Geometry: final body of the model. Coordinates: model frame, mm. A direction names the side the tool comes from. Give positions to 0.01 mm unless a question says otherwise; leave off trailing zeros. Write each loop counter-clockwise with the first axis right and the second up, starting at its lowest first coordinate (ties: lowest second). Pieces come first, ordered by that corner, then holes.
```python
from build123d import *

# Parameters (mm, degrees)
FILLET2_R      = 6
CHAMFER1_SIZE  = 1
CHAMFER1_SIZE2 = 2
CHAMFER2_SIZE  = 0.5


with BuildPart() as part:
    # Sketch1 → Revolve1 (revolve)
    with BuildSketch(Plane(origin=(0, 0, 0), x_dir=(0, 0, -1), z_dir=(1, 0, 0))):
        Polygon((0, 0), (0, -80), (11, -80), (11, -77), (2.5, -77), (2.5, -8), (1.5, -8), (1.5, -3), (2.5, -3), (2.5, 0), align=None)
    revolve(axis=Axis((0, 0, 0), (0, -1, 0)))

    # Fillet2
    fillet2_edges = [part.edges().sort_by_distance(p)[0] for p in [
        (0, -77, 2.5),
    ]]
    fillet(fillet2_edges, radius=FILLET2_R)

    # Chamfer1
    chamfer1_edges = [part.edges().sort_by_distance(p)[0] for p in [
        (0, -77, 11),
    ]]
    chamfer1_side = [part.faces().sort_by_distance(p)[0] for p in [
        (0, -78.5, 11),
    ]]
    chamfer(chamfer1_edges, length=CHAMFER1_SIZE, length2=CHAMFER1_SIZE2, reference=chamfer1_side[0])

    # Chamfer2
    chamfer2_edges = [part.edges().sort_by_distance(p)[0] for p in [
        (0, 0, 2.5),
    ]]
    chamfer(chamfer2_edges, length=CHAMFER2_SIZE)


solid = part.part
```
Item 1: Pull-direction query (Y, two-part tool) for faces 4 (the face through (0, -3, 2)), 5 (the face through (-2.44, -1.73, 0.54)), 6 (the face through (0, 0, 0)); classes: +Y half, -Y half, draft (parallel to the pull), parting line (faces both ways), or undercut.
Found:
face 4: undercut
face 5: draft
face 6: +Y half
Item 2: Section A-A, the plane x = 0. Return the cut outline in (y, z).
Found:
outline: (-80, -11) - (-78, -11) - (-77, -9) - (-77, -8.5) arc R6 cw to (-71, -2.5) - (-8, -2.5) - (-8, -1.5) - (-3, -1.5) - (-3, -2.5) - (-0.5, -2.5) - (0, -2) - (0, 2) - (-0.5, 2.5) - (-3, 2.5) - (-3, 1.5) - (-8, 1.5) - (-8, 2.5) - (-71, 2.5) arc R6 cw to (-77, 8.5) - (-77, 9) - (-78, 11) - (-80, 11) - close
Item 3: Line query: L1, parallel to X at y = -17.5, z = -2; L2, parallel to Y at x = -8.5, z = -2.5; L3, parallel to X at y = -41.5, z = 1.5. Output: solid intervals per line, ascending.
Found:
L1: x = -1.5 to 1.5
L2: y = -80 to -77
L3: x = -2 to 2
Item 4: Section B-B, the plane z = 0. Return the cut outline in (x, y), plus the area to 3 significant figures.
Found:
outline: (-11, -80) - (11, -80) - (11, -78) - (9, -77) - (8.5, -77) arc R6 cw to (2.5, -71) - (2.5, -8) - (1.5, -8) - (1.5, -3) - (2.5, -3) - (2.5, -0.5) - (2, 0) - (-2, 0) - (-2.5, -0.5) - (-2.5, -3) - (-1.5, -3) - (-1.5, -8) - (-2.5, -8) - (-2.5, -71) arc R6 cw to (-8.5, -77) - (-9, -77) - (-11, -78) - close
area: 454 mm2
Item 5: Section C-C, the plane y = -13.5. Return the cut outline in (x, z), plus the area to 3 significant figures.
Found:
outline: circle Ø5 at (0, 0)
area: 19.6 mm2
Item 6: Reachability of faces 1 (the face through (-3.3, -77, -8)), 2 (the face through (0.07, -5.46, 1.5)), 3 (the face through (0, -80, 0)) from +Z, -Z, +X, -X, +Y, -Y: full face, straight path, thin tool, end or side. Return the list, or none.
Found:
face 1: +Y
face 2: none
face 3: +Z, -Z, +X, -X, -Y
Item 7: Pin query (flat end, axial travel): pin 1 Ø5 at (y, z) = (-12, -4.5) entering from +X. Return the tip coordinate at first contact, or that it passes through.
Found:
pin 1: stops at x = 1.5
